Verification items for the finished model (mm, model axes). Face numbers are marked on the shaded views. A direction names the side the tool comes from. Give positions to 0.01 mm unless a question says otherwise; leave off trailing zeros. Loops run counter-clockwise (first coordinate to the right, second up) from the corner with the lowest first, then second, coordinate; pieces in that order, holes last. Notation, with made-up numbers: M 36,74 L 65,74 A35 ccw 65,109 Z; hole C 79,63.25 d6. An arc over 180 degrees is marked long. Answer in a Markdown table with one row per item.
```python
from build123d import *

# Parameters (mm, degrees)
CONE008_ROLL_ANGLE           = -35.5
BOX001027045032_W            = 10
BOX001027045032_H            = 24
BOX001027045032_DEPTH        = 22
BOX001027045032_ROLL_ANGLE   = -35.5
BOX001027045031_W            = 10
BOX001027045031_H            = 24
BOX001027045031_DEPTH        = 22
TORUS007_R                   = 1.1
TORUS007_PITCH_ANGLE         = 90
CYLINDER137_R                = 4
CYLINDER137_DEPTH            = 6
CYLINDER137_ROLL_ANGLE       = -40
CYLINDER136_R                = 2.2
CYLINDER136_DEPTH            = 10
CYLINDER136_ROLL_ANGLE       = -40
FUSION112047_PLACEMENT_ANGLE = 180


with BuildPart() as cone008:
    # Cone008 → Cone008 (revolve)
    with BuildSketch(Plane.XZ):
        Polygon((0, 0), (1.1, 0), (1.3, 2), (0, 2), align=None)
    revolve(axis=Axis((0, 0, 0), (0, 0, 1)))


with BuildPart() as cone008_1:
    # Cone008 roll: moved
    add(cone008.part.rotate(Axis((0, 0, 0), (1, 0, 0)), CONE008_ROLL_ANGLE))


with BuildPart() as cone008_2:
    # Cone008 placement: moved
    add(cone008_1.part.moved(Location((0, 3.71769, 11.614059))))


with BuildPart() as cube085:
    # Box001027045032 → Box001027045032 (new body)
    with BuildSketch(Plane.XY):
        with Locations((5, 12)):
            Rectangle(BOX001027045032_W, BOX001027045032_H)
    extrude(amount=BOX001027045032_DEPTH)


with BuildPart() as cube085_1:
    # Box001027045032 roll: moved
    add(cube085.part.rotate(Axis((0, 0, 0), (1, 0, 0)), BOX001027045032_ROLL_ANGLE))


with BuildPart() as cube085_2:
    # Box001027045032 placement: moved
    add(cube085_1.part.moved(Location((-5, 0.461228, 13.936871))))


with BuildPart() as cube084:
    # Box001027045031 → Box001027045031 (new body)
    with BuildSketch(Plane(origin=(-5, -4, 0), x_dir=(1, 0, 0), z_dir=(0, 0, 1))):
        with Locations((5, 12)):
            Rectangle(BOX001027045031_W, BOX001027045031_H)
    extrude(amount=BOX001027045031_DEPTH)


with BuildPart() as cut074:
    # Torus007 → Torus007 (revolve)
    with BuildSketch(Plane.XZ):
        with Locations((20, 0)):
            Circle(TORUS007_R)
    revolve(axis=Axis((0, 0, 0), (0, 0, 1)))


with BuildPart() as cut074_1:
    # Torus007 pitch: moved
    add(cut074.part.rotate(Axis((0, 0, 0), (0, 1, 0)), TORUS007_PITCH_ANGLE))


with BuildPart() as cut074_2:
    # Torus007 placement: moved
    add(cut074_1.part.moved(Location((0, 20, 0))))

    # Common059: intersect Cube084
    add(cube084.part, mode=Mode.INTERSECT)

    # Cut074: cut Cube085
    add(cube085_2.part, mode=Mode.SUBTRACT)


with BuildPart() as cylinder195:
    # Cylinder137 → Cylinder137 (new body)
    with BuildSketch(Plane.XY):
        Circle(CYLINDER137_R)
    extrude(amount=CYLINDER137_DEPTH)


with BuildPart() as cylinder195_1:
    # Cylinder137 roll: moved
    add(cylinder195.part.rotate(Axis((0, 0, 0), (1, 0, 0)), CYLINDER137_ROLL_ANGLE))


with BuildPart() as cylinder195_2:
    # Cylinder137 placement: moved
    add(cylinder195_1.part.moved(Location((0, 7.571655, 16.302952))))


with BuildPart() as obj1:
    # Cylinder136 → Cylinder136 (new body)
    with BuildSketch(Plane.XY):
        Circle(CYLINDER136_R)
    extrude(amount=CYLINDER136_DEPTH)


with BuildPart() as obj1_1:
    # Cylinder136 roll: moved
    add(obj1.part.rotate(Axis((0, 0, 0), (1, 0, 0)), CYLINDER136_ROLL_ANGLE))


with BuildPart() as obj1_2:
    # Cylinder136 placement: moved
    add(obj1_1.part.moved(Location((0, 4.679111, 12.855752))))

    # Fusion112047: union Cone008, Cut074, Cylinder195
    add(cone008_2.part)
    add(cut074_2.part)
    add(cylinder195_2.part)


with BuildPart() as obj1_3:
    # Fusion112047 placement: moved
    add(obj1_2.part.moved(Location((0, 0, 11))).rotate(Axis((0, 0, 11), (0, 0, 1)), FUSION112047_PLACEMENT_ANGLE))


solid = obj1_3.part
```
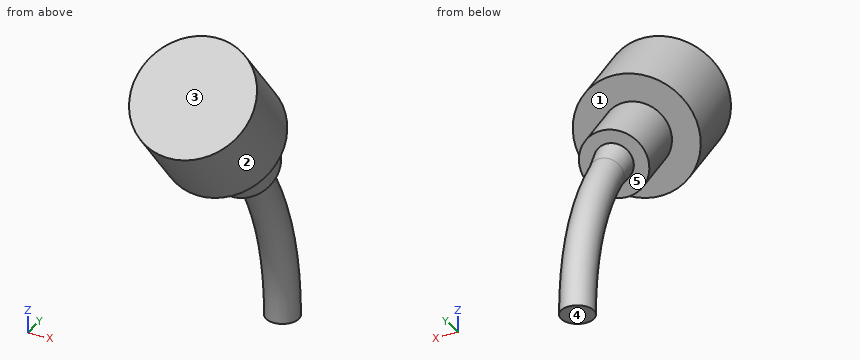
Item 1: Sectioned sample at C-C (x = 3.25). Record the cut outline in (y, z), and give its area (3 significant figures).
Reported:
| item | result |
|---|---|
| outline | M -13.21,30.4 L -9.36,25.8 L -5.79,28.8 L -9.64,33.4 Z |
| area | 28.0 mm^2 |
Item 2: Tool access check on the marked faces 4 and 5. Record the directions out of +Z, -Z, +X, -X, +Y, -Y that give a thin tool (end or side, any length) a straight path to the whole face; none if there is none.
Reported:
| item | result |
|---|---|
| face 4 | -Z, +X, -X, +Y, -Y |
| face 5 | none |
Item 3: Sectioned sample at A-A (x = 1.75). Record the cut outline in (y, z).
Reported:
| item | result |
|---|---|
| outline | M -14.18,29.59 L -10.33,24.99 L -8.59,26.45 L -5.7,23 L -3.66,24.71 L -6.55,28.16 L -4.82,29.61 L -8.67,34.21 Z |
Item 4: Sectioned sample at B-B (x = -3). Record the cut outline in (y, z), and give its area (3 significant figures).
Reported:
| item | result |
|---|---|
| outline | M -13.46,30.2 L -9.6,25.6 L -5.54,29 L -9.4,33.6 Z |
| area | 31.7 mm^2 |
Item 5: Go/stop test with flat-tipped pins: pin 1 (1 mm diameter, centred on x = 1.5, z = 28, fed in from -Y); pin 2 (2 mm diameter, centred on y = -4.5, z = 22, fed in from +X); pin 3 (8 mm diameter, centred on y = -8, z = 27, fed in from +X). Record where each tip stops, or that it passes through.
Reported:
| item | result |
|---|---|
| pin 1 | stops at y = -13.48 |
| pin 2 | stops at x = 1.14 |
| pin 3 | stops at x = 4 |
Item 6: Scan lines: L1, parallel to X at y = -8.75, z = 29; L2, parallel to Y at x = 0.5, z = 18.5; L3, parallel to Z at x = -2.75, y = -13.25. Record each from-to range of solid material in increasing order. Write a range as [from, to].
Reported:
| item | result |
|---|---|
| L1 | x = [-4, 4] |
| L2 | y = [-2.52, -0.41] |
| L3 | z = [29.55, 30.37] |
Item 7: Release check for a two-part mould opening along Y. For the marked faces 1, 2 and 3 record: released by +Y, released by -Y, zero draft, split by the parting line, or undercut.
Reported:
| item | result |
|---|---|
| face 1 | undercut |
| face 2 | split by the parting line |
| face 3 | released by -Y |
